from build123d import *

# Parameters (mm, degrees)
SKETCH1_W           = 111
SKETCH1_H           = 30.5
BOSS_EXTRUDE1_DEPTH = 2
SKETCH2_R           = 0.75
SKETCH2_R_2         = 9
SKETCH2_W           = 25.5
SKETCH2_H           = 10.5
CUT_EXTRUDE1_DEPTH  = 116.131446616
FILLET1_R           = 1
FILLET2_R           = 2


with BuildPart() as part:
    # Sketch1 → Boss-Extrude1 (new body)
    with BuildSketch(Plane(origin=(0, 0, 0), x_dir=(1, 0, 0), z_dir=(0, 1, 0))):
        with Locations((55.5, 15.25)):
            Rectangle(SKETCH1_W, SKETCH1_H)
    extrude(amount=BOSS_EXTRUDE1_DEPTH)

    # Sketch2 → Cut-Extrude1 (cut, through all)
    with BuildSketch(Plane(origin=(0, 2, 0), x_dir=(1, 0, 0), z_dir=(0, 1, 0))):
        with Locations(Location((2, 28.5, 0), (0, 0, 270))):
            Circle(SKETCH2_R)
        with Locations(Location((2, 2, 0), (0, 0, 270))):
            Circle(SKETCH2_R)
        with Locations(Location((109, 2, 0), (0, 0, 270))):
            Circle(SKETCH2_R)
        with Locations(Location((109, 28.5, 0), (0, 0, 270))):
            Circle(SKETCH2_R)
        with Locations(Location((70.76, 15.31, 0), (0, 0, 270))):
            Circle(SKETCH2_R_2)
        with Locations((93.24, 9.85)):
            Rectangle(SKETCH2_W, SKETCH2_H)
    extrude(amount=-CUT_EXTRUDE1_DEPTH, mode=Mode.SUBTRACT)

    # Fillet1
    fillet1_edges = [part.edges().sort_by_distance(p)[0] for p in [
        (111, 2, -15.25),
        (55.5, 2, -30.5),
        (0, 2, -15.25),
        (55.5, 2, 0),
    ]]
    fillet(fillet1_edges, radius=FILLET1_R)

    # Fillet2
    # the kernel refuses this fillet: 2 mm, written as the material it takes off along each edge
    with BuildSketch(Plane(origin=(109, 2, -2), x_dir=(0, 0, 1), z_dir=(-1, 0, 0))) as fillet2_piece_1:
        with BuildLine():
            CenterArc((1, -1), 1, 0, 90)
            Line((2, -1), (2, 0))
            Line((2, 0), (1, 0))
        make_face()
    revolve(axis=Axis((109, 2, -2), (0, 1, 0)), revolution_arc=90, mode=Mode.SUBTRACT)
    with BuildSketch(Plane(origin=(2, 2, -2), x_dir=(-1, 0, 0), z_dir=(0, 0, -1))) as fillet2_piece_2:
        with BuildLine():
            CenterArc((1, -1), 1, 0, 90)
            Line((2, -1), (2, 0))
            Line((2, 0), (1, 0))
        make_face()
    revolve(axis=Axis((2, 2, -2), (0, 1, 0)), revolution_arc=90, mode=Mode.SUBTRACT)
    with BuildSketch(Plane(origin=(109, 2, -28.5), x_dir=(1, 0, 0), z_dir=(0, 0, 1))) as fillet2_piece_3:
        with BuildLine():
            CenterArc((1, -1), 1, 0, 90)
            Line((2, -1), (2, 0))
            Line((2, 0), (1, 0))
        make_face()
    revolve(axis=Axis((109, 2, -28.5), (0, 1, 0)), revolution_arc=90, mode=Mode.SUBTRACT)
    with BuildSketch(Plane(origin=(2, 2, -28.5), x_dir=(0, 0, -1), z_dir=(1, 0, 0))) as fillet2_piece_4:
        with BuildLine():
            CenterArc((1, -1), 1, 0, 90)
            Line((2, -1), (2, 0))
            Line((2, 0), (1, 0))
        make_face()
    revolve(axis=Axis((2, 2, -28.5), (0, 1, 0)), revolution_arc=90, mode=Mode.SUBTRACT)
    with BuildSketch(Plane(origin=(70.76, 2, -15.31), x_dir=(0, 0, 1), z_dir=(-1, 0, 0))) as fillet2_piece_5:
        with BuildLine():
            CenterArc((9 + FILLET2_R, -FILLET2_R), FILLET2_R, 90, 90)
            Line((9, -FILLET2_R), (9, 0))
            Line((9, 0), (9 + FILLET2_R, 0))
        make_face()
    revolve(axis=Axis((70.76, 2, -15.31), (0, 1, 0)), mode=Mode.SUBTRACT)
    with BuildSketch(Plane(origin=(0, -5, -30.5), x_dir=(0, 0, 1), z_dir=(0, 1, 0)), Plane(origin=(0, -5, 0), x_dir=(1, 0, 0), z_dir=(0, 1, 0))) as fillet2_piece_6:
        with BuildLine():
            CenterArc((FILLET2_R, FILLET2_R), FILLET2_R, 180, 90)
            Line((0, FILLET2_R), (0, 0))
            Line((0, 0), (FILLET2_R, 0))
        make_face()
    extrude(amount=7, mode=Mode.SUBTRACT)
    with BuildSketch(Plane(origin=(111, -5, -30.5), x_dir=(0, 0, 1), z_dir=(0, 1, 0)), Plane(origin=(111, -5, 0), x_dir=(-1, 0, 0), z_dir=(0, 1, 0))) as fillet2_piece_7:
        with BuildLine():
            CenterArc((FILLET2_R, -FILLET2_R), FILLET2_R, 90, 90)
            Line((0, -FILLET2_R), (0, 0))
            Line((0, 0), (FILLET2_R, 0))
        make_face()
    extrude(amount=7, mode=Mode.SUBTRACT)


solid = part.part
CAD build for the part. Positions are in the model's coordinates, mm. A direction names the side the tool comes from. Round coordinates to 2 decimals unless told otherwise and drop trailing zeros. Write each loop counter-clockwise with the first axis right and the second up, starting at its lowest first coordinate (ties: lowest second). Pieces come first, ordered by that corner, then holes. Notation, with made-up numbers: (48.25, -26.5) -> (96.25, -26.5) arc R27 cw to (96.25, -6.5) -> close; hole circle Ø4 at (-34, 8). An arc over 180 degrees is marked (long way). Answer as a JSON object with one key per item and string values.
(1) Probe probe 1 along X at (y, z) = (0.5, -2); probe 2 along Z at (x, y) = (109, 0.9); probe 3 along X at (y, z) = (1.1, -28). List the from-to ranges inside material, lowest first. Write a range as [from, to].
Reported:
{"probe 1": "x = [0, 1.25], [2.75, 108.25], [109.75, 111]", "probe 2": "z = [-30.5, -29.25], [-27.75, -2.75], [-1.25, 0]", "probe 3": "x = [0.01, 1.44], [2.56, 108.44], [109.56, 110.99]"}
(2) Two-plate mould, pull along X, no slides. Class faces 1 (the face through (0.57, 0.49, -0.6)), 2 (the face through (110.43, 0.49, -29.9)), 3 (the face through (93, 1, -4.6)), 4 (the face through (80.49, 1, -10)): +X half, -X half, draft (parallel to the pull), parting line (faces both ways), or undercut.
Reported:
{"face 1": "-X half", "face 2": "+X half", "face 3": "undercut", "face 4": "undercut"}
(3) Band-saw the part on B-B, the plane z = -7.5. Count the separate pieces of the cut face and the enclosed holes in it, then the cut area to 3 significant figures.
Reported:
{"separate pieces": "3", "enclosed holes": "0", "area": "150 mm^2"}
(4) Which spindle directions (+Z, -Z, +X, -X, +Y, -Y) get a long thin tool onto all of the face, cutting with end or side? Do faces 5 (the face through (105.99, 1, -10)), 6 (the face through (43, 2, -15)). Say none if no direction does.
Reported:
{"face 5": "+Y, -Y", "face 6": "+Z, -Z, +X, -X, +Y"}
(5) Band-saw the part on A-A, the plane x = 85.5. List the corners of the cut face in (y, z).
Reported:
{"outline": "(0, -30.5) -> (1, -30.5) arc R1 ccw to (2, -29.5) -> (2, -15.1) -> (0, -15.1) -> close; (0, -4.6) -> (2, -4.6) -> (2, -1) arc R1 ccw to (1, 0) -> (0, 0) -> close"}
(6) Pin check, flat tips, straight feed: P1, Ø4, axis at x = 43.5, z = -9, coming from the -Y side; P2, Ø0.6, axis at y = 1.5, z = -8.5, coming from the +X side; P3, Ø0.6, axis at y = 1.5, z = -8.5, coming from the -X side. Stop position of each tip, or through.
Reported:
{"P1": "stops at y = 0", "P2": "stops at x = 110.98", "P3": "stops at x = 0.02"}
